Geometry check sheet. Reference: the model listing, model coordinates, mm. Face numbers are marked on the shaded views. A direction names the side the tool comes from. Coordinates: 2 decimals unless noted, no trailing zeros. Order: outer loops, then holes, each group sorted by start corner. A loop starts at its lowest first (then second) coordinate and runs counter-clockwise, first axis right, second up. Notation, with made-up numbers: M 40.25,89 L 57.25,89 A13 cw 57.25,104 Z; hole C 35.5,-15 d2. An arc over 180 degrees is marked long. One line per item, written item: value. Start each with the question number.
1) Sectioned sample at D-D, the plane y = 45. Enter the section's corners in (x, z).
2) Sectioned sample at A-A, the plane z = -10. Enter the section's corners in (x, y).
3) Access from +Z, -Z, +X, -X, +Y, -Y to the whole of each face (thin tool, end or side, straight path). Record for the marked faces 1, 2 and 3.
4) Thickness scan on L1, parallel to X at y = 49, z = 0; L2, parallel to Y at x = -2.5, z = -2; L3, parallel to X at y = -10, z = 10.75 (3 decimals). Record the ranges inside material, lowest first. Write a range as from..to.
5) Go/stop test with flat-tipped pins: P1, Ø8, axis at x = -26.5, z = -10, coming from the +Y side; P2, Ø1.4, axis at x = 0.5, z = 0, coming from the +Y side; P3, Ø10, axis at x = -8.5, y = -11.5, coming from the -Z side. Record where each tip stops, or that it passes through.
6) Sectioned sample at B-B, the plane x = -27.73. Enter the section's corners in (y, z).
7) Sectioned sample at C-C, the plane y = 23. Enter the section's corners in (x, z), then the cut area to 3 significant figures.
8) Draft check along Z on the marked faces 4, 5, 6 and 7. Enter one of: pulls with the +Z half, pulls with the -Z half, needs draft (parallel to the pull), parting line crosses it, or undercut.
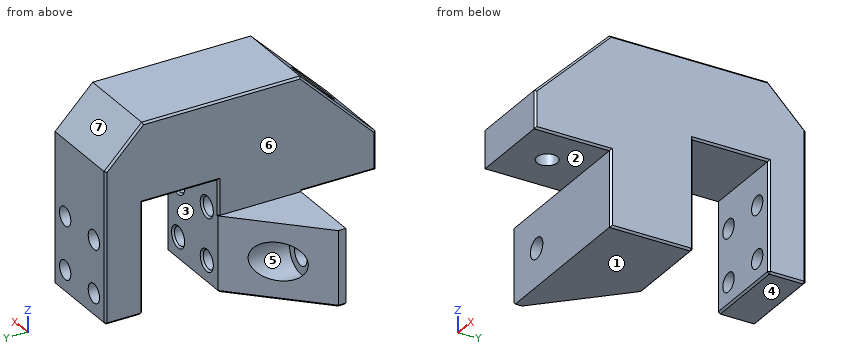
```python
from build123d import *

# Parameters (mm, degrees)
SKETCH2_W                      = 22.73
SKETCH2_H                      = 30
BOSS_EXTRUDE1_DEPTH            = 52
SKETCH3_W                      = 22.73
SKETCH3_H                      = 10
BOSS_EXTRUDE2_DEPTH            = 20
CBORE_FOR_M5_SHCS1_D           = 5.5
CBORE_FOR_M5_SHCS1_CBORE_D     = 10
CBORE_FOR_M5_SHCS1_CBORE_DEPTH = 5
BOSS_EXTRUDE3_START            = 20
SKETCH7_W                      = 22.73
SKETCH7_H                      = 72
SKETCH7_R                      = 5
BOSS_EXTRUDE3_DEPTH            = 20
SKETCH8_W                      = 29.2
SKETCH8_H                      = 20
CUT_EXTRUDE1_DEPTH             = 65.192311845
CUT_EXTRUDE2_REACH             = 81.99
SKETCH9_R                      = 2.5
SKETCH10_R                     = 2.4
CUT_EXTRUDE3_DEPTH             = 20
SKETCH12_W                     = 20
SKETCH12_H                     = 22
BOSS_EXTRUDE5_DEPTH            = 20
CBORE_FOR_M5_SHCS2_D           = 5.5
CBORE_FOR_M5_SHCS2_CBORE_D     = 10
CBORE_FOR_M5_SHCS2_CBORE_DEPTH = 16
CHAMFER1_SIZE                  = 20
CHAMFER3_SIZE                  = 10
CHAMFER2_SIZE                  = 0.5


with BuildPart() as part:
    # Sketch2 → Boss-Extrude1 (new body)
    with BuildSketch(Plane(origin=(0, 0, 0), x_dir=(1, 0, 0), z_dir=(0, 1, 0))):
        with Locations((-6.365, 5)):
            Rectangle(SKETCH2_W, SKETCH2_H)
    extrude(amount=BOSS_EXTRUDE1_DEPTH)

    # Sketch3 → Boss-Extrude2 (add)
    with BuildSketch(Plane.XZ):
        with Locations((-6.365, 5)):
            Rectangle(SKETCH3_W, SKETCH3_H)
    extrude(amount=BOSS_EXTRUDE2_DEPTH)

    # CBORE for M5 SHCS1 (through all)
    with Locations(Plane.XY.offset(10)):
        with Locations((-6.365, -10)):
            CounterBoreHole(CBORE_FOR_M5_SHCS1_D / 2, CBORE_FOR_M5_SHCS1_CBORE_D / 2, CBORE_FOR_M5_SHCS1_CBORE_DEPTH)

    # Sketch7 → Boss-Extrude3 (add)
    with BuildSketch(Plane.XY.offset(10).offset(BOSS_EXTRUDE3_START)):
        with Locations((-6.365, 16)):
            Rectangle(SKETCH7_W, SKETCH7_H)
        with Locations((-6.365, -10)):
            Circle(SKETCH7_R, mode=Mode.SUBTRACT)
    extrude(amount=-BOSS_EXTRUDE3_DEPTH)

    # Sketch8 → Cut-Extrude1 (cut, through all)
    with BuildSketch(Plane(origin=(5, 0, 0), x_dir=(0, 0, -1), z_dir=(1, 0, 0))):
        with Locations((5.4, 32)):
            Rectangle(SKETCH8_W, SKETCH8_H)
    extrude(amount=-CUT_EXTRUDE1_DEPTH, mode=Mode.SUBTRACT)

    # Sketch9 → Cut-Extrude2 (cut, up to next)
    with BuildSketch(Plane(origin=(0, 52, 0), x_dir=(1, 0, 0), z_dir=(0, 1, 0)), mode=Mode.PRIVATE) as cut_extrude2_sk1:
        with Locations(Location((-12.73, 0, 0), (0, 0, 270))):
            Circle(SKETCH9_R)
    cut_extrude2_tool1 = extrude(cut_extrude2_sk1.sketch, amount=-CUT_EXTRUDE2_REACH, mode=Mode.PRIVATE) & part.part
    # Sketch9 → Cut-Extrude2 (cut, up to next)
    with BuildSketch(Plane(origin=(0, 52, 0), x_dir=(1, 0, 0), z_dir=(0, 1, 0)), mode=Mode.PRIVATE) as cut_extrude2_sk2:
        with Locations(Location((0, 14, 0), (0, 0, 270))):
            Circle(SKETCH9_R)
    cut_extrude2_tool2 = extrude(cut_extrude2_sk2.sketch, amount=-CUT_EXTRUDE2_REACH, mode=Mode.PRIVATE) & part.part
    # Sketch9 → Cut-Extrude2 (cut, up to next)
    with BuildSketch(Plane(origin=(0, 52, 0), x_dir=(1, 0, 0), z_dir=(0, 1, 0)), mode=Mode.PRIVATE) as cut_extrude2_sk3:
        with Locations(Location((-12.73, 14, 0), (0, 0, 270))):
            Circle(SKETCH9_R)
    cut_extrude2_tool3 = extrude(cut_extrude2_sk3.sketch, amount=-CUT_EXTRUDE2_REACH, mode=Mode.PRIVATE) & part.part
    # Sketch9 → Cut-Extrude2 (cut, up to next)
    with BuildSketch(Plane(origin=(0, 52, 0), x_dir=(1, 0, 0), z_dir=(0, 1, 0)), mode=Mode.PRIVATE) as cut_extrude2_sk4:
        with Locations(Location((0, 0, 0), (0, 0, 270))):
            Circle(SKETCH9_R)
    cut_extrude2_tool4 = extrude(cut_extrude2_sk4.sketch, amount=-CUT_EXTRUDE2_REACH, mode=Mode.PRIVATE) & part.part
    add(cut_extrude2_tool1.solids().sort_by_distance((-12.73, 52, 0))[0], mode=Mode.SUBTRACT)
    add(cut_extrude2_tool2.solids().sort_by_distance((0, 52, -14))[0], mode=Mode.SUBTRACT)
    add(cut_extrude2_tool3.solids().sort_by_distance((-12.73, 52, -14))[0], mode=Mode.SUBTRACT)
    add(cut_extrude2_tool4.solids().sort_by_distance((0, 52, 0))[0], mode=Mode.SUBTRACT)

    # Sketch10 → Cut-Extrude3 (cut)
    with BuildSketch(Plane(origin=(0, 22, 0), x_dir=(1, 0, 0), z_dir=(0, 1, 0))):
        with Locations(Location((0, 0, 0), (0, 0, 270))):
            Circle(SKETCH10_R)
        with Locations(Location((-12.73, 0, 0), (0, 0, 270))):
            Circle(SKETCH10_R)
        with Locations(Location((-12.73, 14, 0), (0, 0, 270))):
            Circle(SKETCH10_R)
        with Locations(Location((0, 14, 0), (0, 0, 270))):
            Circle(SKETCH10_R)
    extrude(amount=-CUT_EXTRUDE3_DEPTH, mode=Mode.SUBTRACT)

    # Sketch12 → Boss-Extrude5 (add)
    with BuildSketch(Plane(origin=(0, 0, -20), x_dir=(-1, 0, 0), z_dir=(0, 0, -1))):
        with Locations((27.73, 11)):
            Rectangle(SKETCH12_W, SKETCH12_H)
    extrude(amount=-BOSS_EXTRUDE5_DEPTH)

    # CBORE for M5 SHCS2 (through all)
    with Locations(Plane(origin=(0, 22, 0), x_dir=(1, 0, 0), z_dir=(0, 1, 0))):
        with Locations((-27.73, 10)):
            CounterBoreHole(CBORE_FOR_M5_SHCS2_D / 2, CBORE_FOR_M5_SHCS2_CBORE_D / 2, CBORE_FOR_M5_SHCS2_CBORE_DEPTH)

    # Chamfer1
    # the kernel refuses this chamfer: 20 mm, written as the material it takes off along each edge
    with BuildSketch(Plane(origin=(-69.163659759, -20, 30), x_dir=(0, 0.9996219169112968, 0.027495876610586317), z_dir=(1, 0, 0))) as chamfer1_piece_1:
        Polygon((CHAMFER1_SIZE * 0.999621916911, -CHAMFER1_SIZE * 0.0274958766106), (-CHAMFER1_SIZE * 0.0274958766106, -CHAMFER1_SIZE * 0.999621916911), (0, 0), align=None)
    extrude(amount=125.597319519, mode=Mode.SUBTRACT)
    with BuildSketch(Plane(origin=(-37.73, 22, -71.433659759), x_dir=(0.9996219169112968, 0.027495876610586317, 0), z_dir=(0, 0, 1))) as chamfer1_piece_2:
        Polygon((CHAMFER1_SIZE * 0.999621916911, -CHAMFER1_SIZE * 0.0274958766106), (-CHAMFER1_SIZE * 0.0274958766106, -CHAMFER1_SIZE * 0.999621916911), (0, 0), align=None)
    extrude(amount=122.867319519, mode=Mode.SUBTRACT)

    # Chamfer3
    chamfer3_edges = [part.edges().sort_by_distance(p)[0] for p in [
        (-6.365, 52, 30),
    ]]
    chamfer(chamfer3_edges, length=CHAMFER3_SIZE)

    # Chamfer2
    chamfer2_edges = [part.edges().sort_by_distance(p)[0] for p in [
        (5, 52, 0),
        (5, 11, -20),
        (5, 47, -20),
        (5, 0, -10),
        (5, -10, 0),
        (5, -20, 5),
        (5, -10, 20),
        (5, 21, 30),
        (-17.73, -10, 0),
        (-17.73, 47, -20),
        (-17.73, 52, 0),
        (-17.73, 21, 30),
        (-17.73, -10, 20),
        (-17.73, -20, 5),
        (5, 42, -5.4),
        (5, 32, 9.2),
        (5, 22, -5.4),
        (-17.73, 22, 4.6),
        (-17.73, 32, 9.2),
        (-17.73, 42, -5.4),
        (0, 22, -16.4),
        (-12.73, 22, -16.4),
        (-12.73, 22, -2.4),
        (0, 22, -2.4),
        (5, 47, 25),
        (-17.73, 47, 25),
        (-37.73, 1, -20),
        (-27.73, 12, -20),
        (-6.365, 22, -20),
        (-6.365, 42, -20),
        (-6.365, 52, -20),
    ]]
    chamfer(chamfer2_edges, length=CHAMFER2_SIZE)


solid = part.part
```
Final values:
1. outline: M -17.73,-19.5 L -17.23,-20 L 4.5,-20 L 5,-19.5 L 5,26.29 L 4.5,27 L -17.23,27 L -17.73,26.29 Z; hole C -12.73,-14 d5; hole C -12.73,0 d5; hole C 0,-14 d5; hole C 0,0 d5
2. outline: M -37.73,0 L -30.48,0 L -30.48,6 L -32.73,6 L -32.73,7 L -37.73,2 Z; M -24.98,0 L 4.5,0 L 5,0.5 L 5,21.5 L 4.5,22 L -17.73,22 L -22.73,17 L -22.73,6 L -24.98,6 Z; M -17.73,42.5 L -17.23,42 L 4.5,42 L 5,42.5 L 5,51.5 L 4.5,52 L -17.23,52 L -17.73,51.5 Z
3. face 1: -Z, +X, -X, +Y, -Y
3. face 2: -Z, +X, -X, -Y
3. face 3: -Z, +X, -X
4. L1: x = -17.73..-15.23, -10.23..-2.5, 2.5..5
4. L2: y = 0..22, 42..52
4. L3: x = -17.73..-11.365, -1.365..5
5. P1: stops at y = 17.23
5. P2: stops at y = 2
5. P3: stops at z = 0
6. outline: M 0,-20 L 11.29,-20 L 12,-19.5 L 12,-15 L 6,-15 L 6,-12.75 L 0,-12.75 Z; M 0,-7.25 L 6,-7.25 L 6,-5 L 12,-5 L 12,0 L 0,0 Z
7. outline: M -17.73,9.7 L -17.23,9.2 L 4.5,9.2 L 5,9.7 L 5,29.5 L 4.5,30 L -17.23,30 L -17.73,29.5 Z
7. area: 472 mm^2
8. face 4: pulls with the -Z half
8. face 5: undercut
8. face 6: needs draft
8. face 7: pulls with the +Z half
